from build123d import *

# Parameters (mm, degrees)
F0_R     = 10
F1_DEPTH = 2.5
F2_R     = 2
F4_R     = 3
F5_DEPTH = 25


with BuildPart() as f1:
    # F0 (on Top) → F1 (new body, symmetric)
    with BuildSketch(Plane.XY):
        Circle(F0_R)
    extrude(amount=F1_DEPTH, both=True)

    # F2 (on Right) → F3 (revolve, cut)
    with BuildSketch(Plane.YZ):
        with Locations((10, 0)):
            Circle(F2_R)
    revolve(axis=Axis((0, 0, 4.383557), (0, 0, 1)), mode=Mode.SUBTRACT)

    # F4 (on face) → F5 (cut)
    with BuildSketch(Plane.XY.offset(2.5)):
        Circle(F4_R)
    extrude(amount=-F5_DEPTH, mode=Mode.SUBTRACT)


solid = f1.part
The listing builds one solid part. Answer for the finished solid, in the listing's coordinates (mm). Round coordinates to 2 decimals unless told otherwise and drop trailing zeros. Loops run counter-clockwise (first coordinate to the right, second up) from the corner with the lowest first, then second, coordinate; pieces in that order, holes last. Notation, with made-up numbers: M 5,3 L 44,3 A23 ccw 44,38 Z; hole C -28,-12.5 d1. An arc over 180 degrees is marked long. Write each question's results on one line, items separated by ' | '. Start each with the question number.
1) Determine the mould class of faces 1 (the cylindrical face through (-3, 0, 0)), 2 (the flat face through (2.1, 2.4, 2.5)), 3 (the cylindrical face through (5.38, 8.43, 2.25)) for opening direction X: pulls with the +X half, pulls with the -X half, needs draft (parallel to the pull), parting line crosses it, or undercut.
2) Straight lines are drawn through the part: probe 1 along Z at (x, y) = (-6.5, -6.75); probe 2 along Y at (x, z) = (0, 0.3); probe 3 along Y at (x, z) = (0, -1.45). For each, find the intervals that lie inside material, in ascending order.
3) Find section C-C on z = -1.55. Write down the section's boundary in (x, y).
4) Find section D-D on z = 0.1. Write down the section's boundary in (x, y) (1 decimal), plus the area to 3 significant figures.
5) Find section A-A on x = 0. Write down the section's boundary in (y, z), plus the area to 3 significant figures.
6) Each of these flat-tipped pins is pushed along its axis until it touches: pin 1 (3 mm diameter, centred on x = 7.5, z = 0, fed in from -Y); pin 2 (1 mm diameter, centred on x = -2.5, z = 0.5, fed in from -Y); pin 3 (1.5 mm diameter, centred on x = 1, z = -2, fed in from +Y). Where does it stop, or does it pass through?
Final values:
1) face 1: undercut | face 2: needs draft | face 3: parting line crosses it
2) probe 1: -2.5 to -1.9, 1.9 to 2.5 | probe 2: -8.02 to -3, 3 to 8.02 | probe 3: -8.62 to -3, 3 to 8.62
3) outline: C 0,0 d17.47; hole C 0,0 d6
4) outline: C 0,0 d16; hole C 0,0 d6 | area: 173 mm²
5) outline: M -10,-2.5 L -3,-2.5 L -3,2.5 L -10,2.5 L -10,2 A2 cw -10,-2 Z; M 3,-2.5 L 10,-2.5 L 10,-2 A2 cw 10,2 L 10,2.5 L 3,2.5 Z | area: 57.4 mm²
6) pin 1: y = -5.29 | pin 2: y = -7.92 | pin 3: y = 10
